Input: part model. Units: mm. Frame: model coordinates. Face numbers are marked on the shaded views. A direction names the side the tool comes from. Give positions to 0.01 mm unless a question says otherwise; leave off trailing zeros. Order: outer loops, then holes, each group sorted by start corner. A loop starts at its lowest first (then second) coordinate and runs counter-clockwise, first axis right, second up. Notation, with made-up numbers: (62, 60) - (112, 60) arc R21 cw to (112, 81) - close; hole circle Ø7 at (-35.5, -23). An arc over 180 degrees is marked (long way). Answer in a Markdown table with one row per item. Add a question column.
1. Section query C-C on z = 6.5. Return loops of the section in (x, y), and give its area (3 significant figures).
2. Section query B-B on x = 4.75. Return loops of the section in (y, z), and give its area (3 significant figures).
3. Section query D-D on y = -1.5. Return loops of the section in (x, z).
4. Access query for the marked faces 4, 5 and 6. Directions: +Z, -Z, +X, -X, +Y, -Y. A direction counts if a zero-diameter tool reaches every point of the face in a straight line with its end or side. Return the directions, or none.
5. Contact query for flat-ended pins moving along their axis: pin 1 (1.2 mm diameter, centred on x = -5.5, z = 5.5, fed in from -Y); pin 2 (5 mm diameter, centred on x = 0, y = 6.5, fed in from +Z); pin 3 (3 mm diameter, centred on x = -4.75, y = 7.5, fed in from -Z); pin 4 (1 mm diameter, centred on x = -1.5, z = 5.5, fed in from -Y). Output: stop coordinate, or through.
6. Section query A-A on y = 7.5. Return loops of the section in (x, z), and give its area (3 significant figures).
7. Mould query, pull axis Y, two halves, no side actions, for the marked faces 1, 2 and 3. Classes: released by +Y, released by -Y, zero draft, split by the parting line, or undercut.
8. Ray query, line 1 (Y direction, x = -4.75, z = 1); line 2 (X direction, y = 1.25, z = 1); line 3 (Y direction, x = -4.75, z = 3.5). Return the intervals inside material, ascending. Write a range as [from, to].
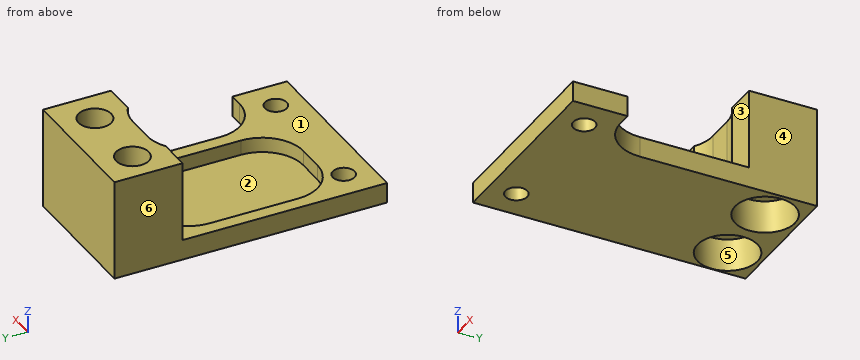
```python
from build123d import *

# Parameters (mm, degrees)
SKETCH1_W                                           = 14
SKETCH1_H                                           = 20
BOSS_EXTRUDE1_DEPTH                                 = 1.5
SKETCH2_W                                           = 14
SKETCH2_H                                           = 5
BOSS_EXTRUDE2_DEPTH                                 = 5.9
M2_TAPPED_HOLE1_D                                   = 1.6
M2_TAPPED_HOLE1_DEPTH                               = 6
M2_TAPPED_HOLE1_TIP                                 = 0.480688495
CUT_EXTRUDE6_DEPTH                                  = 15.274452704
CBORE_FOR_M2_HEX_SOCKET_HEAD_CAP_SCREW1_D           = 2.4
CBORE_FOR_M2_HEX_SOCKET_HEAD_CAP_SCREW1_DEPTH       = 7.5
CBORE_FOR_M2_HEX_SOCKET_HEAD_CAP_SCREW1_CBORE_D     = 4.4
CBORE_FOR_M2_HEX_SOCKET_HEAD_CAP_SCREW1_CBORE_DEPTH = 2.4
CBORE_FOR_M2_HEX_SOCKET_HEAD_CAP_SCREW1_TIP         = 0.721032743
CUT_EXTRUDE7_DEPTH                                  = 7


with BuildPart() as part:
    # Sketch1 → Boss-Extrude1 (new body)
    with BuildSketch(Plane.XY):
        Rectangle(SKETCH1_W, SKETCH1_H)
    extrude(amount=BOSS_EXTRUDE1_DEPTH)

    # Sketch2 → Boss-Extrude2 (add)
    with BuildSketch(Plane.XY.offset(1.5)):
        with Locations((0, 7.5)):
            Rectangle(SKETCH2_W, SKETCH2_H)
    extrude(amount=BOSS_EXTRUDE2_DEPTH)

    # M2 Tapped Hole1
    with Locations(Plane(origin=(-4.75, -8, 0), x_dir=(-1, 0, 0), z_dir=(0, 0, -1))):
        with Locations((0, 0), (-9.5, 0)):
            Hole(M2_TAPPED_HOLE1_D / 2, depth=M2_TAPPED_HOLE1_DEPTH)
            with Locations((0, 0, -(M2_TAPPED_HOLE1_DEPTH + M2_TAPPED_HOLE1_TIP / 2))):  # 118° drill point
                Cone(0, M2_TAPPED_HOLE1_D / 2, M2_TAPPED_HOLE1_TIP, mode=Mode.SUBTRACT)

    # Sketch11 → Cut-Extrude6 (cut, through all)
    with BuildSketch(Plane.XY.offset(7.4)):
        with BuildLine():
            Line((7, -6), (6, -6))
            ThreePointArc((6, -6), (3.878679656, -5.121320344), (3, -3))
            Line((3, -3), (3, 10))
            Line((3, 10), (7, 10))
            Line((7, 10), (7, -6))
        make_face()
    extrude(amount=-CUT_EXTRUDE6_DEPTH, mode=Mode.SUBTRACT)

    # CBORE for M2 Hex Socket Head Cap Screw1
    with Locations(Plane(origin=(-4.75, 7.5, 0), x_dir=(-1, 0, 0), z_dir=(0, 0, -1))):
        with Locations((0, 0), (-5.25, 0)):
            CounterBoreHole(CBORE_FOR_M2_HEX_SOCKET_HEAD_CAP_SCREW1_D / 2, CBORE_FOR_M2_HEX_SOCKET_HEAD_CAP_SCREW1_CBORE_D / 2, CBORE_FOR_M2_HEX_SOCKET_HEAD_CAP_SCREW1_CBORE_DEPTH, depth=CBORE_FOR_M2_HEX_SOCKET_HEAD_CAP_SCREW1_DEPTH)
            with Locations((0, 0, -(CBORE_FOR_M2_HEX_SOCKET_HEAD_CAP_SCREW1_DEPTH + CBORE_FOR_M2_HEX_SOCKET_HEAD_CAP_SCREW1_TIP / 2))):  # 118° drill point
                Cone(0, CBORE_FOR_M2_HEX_SOCKET_HEAD_CAP_SCREW1_D / 2, CBORE_FOR_M2_HEX_SOCKET_HEAD_CAP_SCREW1_TIP, mode=Mode.SUBTRACT)

    # Sketch14 → Cut-Extrude7 (cut)
    with BuildSketch(Plane.XY.offset(7.4)):
        with BuildLine():
            Line((-3, 5.5), (-1, 5.5))
            ThreePointArc((-1, 5.5), (1.121320344, 4.621320344), (2, 2.5))
            Line((2, 2.5), (2, -4))
            ThreePointArc((2, -4), (1.121320344, -6.121320344), (-1, -7))
            Line((-1, -7), (-3, -7))
            ThreePointArc((-3, -7), (-5.121320344, -6.121320344), (-6, -4))
            Line((-6, -4), (-6, 2.5))
            ThreePointArc((-6, 2.5), (-5.121320344, 4.621320344), (-3, 5.5))
        make_face()
    extrude(amount=-CUT_EXTRUDE7_DEPTH, mode=Mode.SUBTRACT)


solid = part.part
```
Answer:
| question | item | result |
|---|---|---|
| 1 | outline | (-7, 5) - (-4.66, 5) arc R3 cw to (-3, 5.5) - (-1, 5.5) arc R3 cw to (0.66, 5) - (3, 5) - (3, 10) - (-7, 10) - close; hole circle Ø2.4 at (-4.75, 7.5); hole circle Ø2.4 at (0.5, 7.5) |
| 1 | area | 38.8 mm² |
| 2 | outline | (-10, 0) - (-8.8, 0) - (-8.8, 1.5) - (-10, 1.5) - close; (-7.2, 0) - (-5.73, 0) - (-5.73, 1.5) - (-7.2, 1.5) - close |
| 2 | area | 4.01 mm² |
| 3 | outline | (-7, 0) - (3, 0) - (3, 1.5) - (2, 1.5) - (2, 0.4) - (-6, 0.4) - (-6, 1.5) - (-7, 1.5) - close |
| 4 | face 4 | +Z, -Z, +X, +Y |
| 4 | face 5 | -Z |
| 4 | face 6 | +Z, -Z, -X, +Y, -Y |
| 5 | pin 1 | stops at y = 5 |
| 5 | pin 2 | stops at z = 7.4 |
| 5 | pin 3 | stops at z = 2.4 |
| 5 | pin 4 | stops at y = 5.5 |
| 6 | outline | (-7, 0) - (-6.95, 0) - (-6.95, 2.4) - (-5.95, 2.4) - (-5.95, 7.4) - (-7, 7.4) - close; (-3.55, 2.4) - (-2.55, 2.4) - (-2.55, 0) - (-1.7, 0) - (-1.7, 2.4) - (-0.7, 2.4) - (-0.7, 7.4) - (-3.55, 7.4) - close; (1.7, 2.4) - (2.7, 2.4) - (2.7, 0) - (3, 0) - (3, 7.4) - (1.7, 7.4) - close |
| 6 | area | 28.9 mm² |
| 7 | face 1 | zero draft |
| 7 | face 2 | undercut |
| 7 | face 3 | released by -Y |
| 8 | line 1 | y = [-10, -8.8], [-7.2, -6.44], [4.94, 5.3], [9.7, 10] |
| 8 | line 2 | x = [-7, -6], [2, 3] |
| 8 | line 3 | y = [5, 6.3], [8.7, 10] |
